from build123d import *

# Parameters (mm, degrees)
BOSS_EXTRUDE1_DEPTH     = 304.8
CUT_EXTRUDE2_DEPTH      = 385.371747141
CUT_EXTRUDE2_DEPTH_BACK = 385.371747141
SHELL1_T                = -12.7


with BuildPart() as part:
    # Sketch1 → Boss-Extrude1 (new, symmetric)
    with BuildSketch(Plane.XY):
        Polygon((-101.6, 0), (101.6, 0), (152.4, 50.8), (152.4, 177.8), (-152.4, 177.8), (-152.4, 50.8), align=None)
    extrude(amount=BOSS_EXTRUDE1_DEPTH, both=True)

    # Sketch3 → Cut-Extrude2 (cut, two sides: drawn at the far end of the back side and taken through both)
    with BuildSketch(Plane(origin=(0, 0, 0), x_dir=(0, 0, -1), z_dir=(1, 0, 0)).offset(-CUT_EXTRUDE2_DEPTH_BACK)):
        Polygon((-304.8, 50.8), (-304.8, 0), (-254, 0), align=None)
        Polygon((304.8, 50.8), (304.8, 0), (254, 0), align=None)
    extrude(amount=CUT_EXTRUDE2_DEPTH + CUT_EXTRUDE2_DEPTH_BACK, mode=Mode.SUBTRACT)

    # Shell1
    shell1_openings = [part.faces().sort_by_distance(p)[0] for p in [
        (0, 177.8, 0),
    ]]
    offset(amount=SHELL1_T, openings=shell1_openings, kind=Kind.INTERSECTION)


solid = part.part
Read the model definition and answer for the solid it produces. Units are mm, in the model's axes. A direction names the side the tool comes from. Give positions to 0.01 mm unless a question says otherwise; leave off trailing zeros. Loops run counter-clockwise (first coordinate to the right, second up) from the corner with the lowest first, then second, coordinate; pieces in that order, holes last. Notation, with made-up numbers: (15, 59) - (72, 59) arc R19 ccw to (72, 93) - close; hole circle Ø11 at (21.25, -5.5). An arc over 180 degrees is marked (long way). Answer as CSV lines item,"result". Start each with the question number.
1) Which of the six approach directions +Z, -Z, +X, -X, +Y, -Y give full straight-line access (tool end or side, diameter ignored) to faces 1 (the face through (117.72, 34.08, 4.09)), 2 (the face through (126.6, 25, 4.3))?
2) Determine the mould class of faces 3 (the face through (-2, 25, 279)), 4 (the face through (-1.96, 34.08, -270.12)), 5 (the face through (-127.4, 25.8, 4.3)), 6 (the face through (-2, 118, -292.1)) for opening direction X: released by +X, released by -X, zero draft, split by the parting line, or undercut.
3) Find section C-C (z = -47). Write down the section's boundary in (x, y), then the cut area to 3 significant figures.
4) Find section B-B (x = -78). Write down the section's boundary in (y, z), then the cut area to 3 significant figures.
5) Find section A-A (y = 101). Write down the section's boundary in (x, z), then the cut area to 3 significant figures.
6) This flat-tipped pin is pushed along its axis until it touches: pin 1 Ø12 at (y, z) = (35.5, -59) entering from -X. Where does it stop, or does it pass through?
7) Straight lines are drawn through the part: L1, parallel to Z at x = 90.5, y = 169; L2, parallel to X at y = 124, z = 84; L3, parallel to X at y = 49.5, z = 203.5. For each, find the intervals that lie inside material, in ascending order. Write a range as from..to.
Findings below:
1,face 1,"+Y"
1,face 2,"+Z, -Z, +X, -Y"
2,face 3,"zero draft"
2,face 4,"undercut"
2,face 5,"released by -X"
2,face 6,"undercut"
3,outline,"(-152.4, 50.8) - (-101.6, 0) - (101.6, 0) - (152.4, 50.8) - (152.4, 177.8) - (139.7, 177.8) - (139.7, 56.06) - (96.34, 12.7) - (-96.34, 12.7) - (-139.7, 56.06) - (-139.7, 177.8) - (-152.4, 177.8) - close"
3,area,"7,360 mm^2"
4,outline,"(0, -254) - (50.8, -304.8) - (177.8, -304.8) - (177.8, -292.1) - (56.06, -292.1) - (12.7, -248.74) - (12.7, 248.74) - (56.06, 292.1) - (177.8, 292.1) - (177.8, 304.8) - (50.8, 304.8) - (0, 254) - close"
4,area,"11,200 mm^2"
5,outline,"(-152.4, -304.8) - (152.4, -304.8) - (152.4, 304.8) - (-152.4, 304.8) - close; hole (-139.7, -292.1) - (139.7, -292.1) - (139.7, 292.1) - (-139.7, 292.1) - close"
5,area,"22,600 mm^2"
6,pin 1,"x = -143.1"
7,L1,"-304.8..-292.1, 292.1..304.8"
7,L2,"-152.4..-139.7, 139.7..152.4"
7,L3,"-151.1..-133.14, 133.14..151.1"
